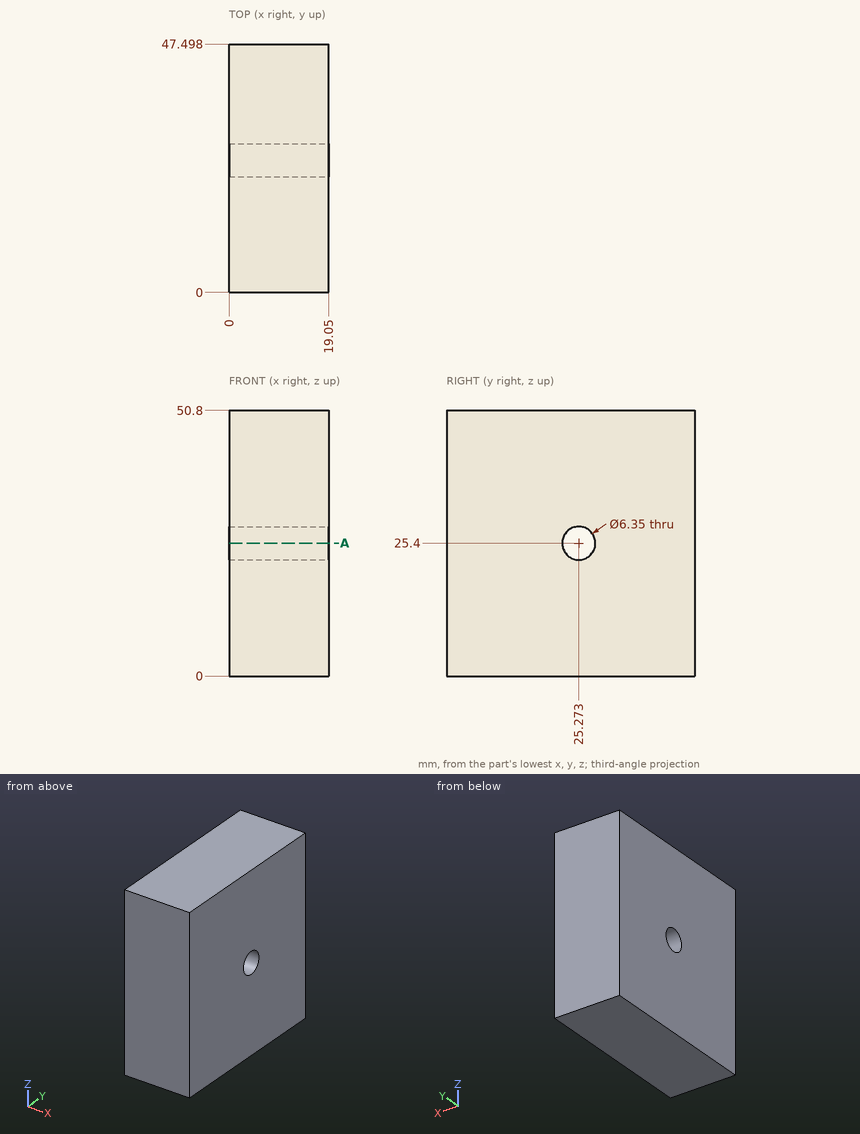
Job drawing, mm, ordinate dimensions from the low corner. One solid piece. Round coordinates to 2 decimals unless told otherwise and drop trailing zeros. Loops run counter-clockwise (first coordinate to the right, second up) from the corner with the lowest first, then second, coordinate; pieces in that order, holes last.
Item 1: Cut at A-A, the plane z = 25.4. Give the cut face in (x, y).
Item 2: Drop a flat-ended pin along its axis: P1, Ø7.5, axis at y = 25.273, z = 25.4, coming from the -X side. Give the stop position or say it passes through.
Item 3: Drill centre lines: line 1 (Y direction, x = 6.5, z = 25.4); line 2 (Z direction, x = 15.5, y = 25); line 3 (Z direction, x = 7.5, y = 23.5). Where is each one in solid material? Low to high.
A:
1. outline: (0, 0) - (19.05, 0) - (19.05, 22.1) - (0, 22.1) - close; (0, 28.45) - (19.05, 28.45) - (19.05, 47.5) - (0, 47.5) - close
2. P1: stops at x = 0
3. line 1: y = 0 to 22.1, 28.45 to 47.5
3. line 2: z = 0 to 22.24, 28.56 to 50.8
3. line 3: z = 0 to 22.77, 28.03 to 50.8
